Work out the finished part from the listing and answer in its coordinate system (mm). A direction names the side the tool comes from. Coordinates: 2 decimals unless noted, no trailing zeros. Order: outer loops, then holes, each group sorted by start corner. A loop starts at its lowest first (then second) coordinate and runs counter-clockwise, first axis right, second up.
1. A tool of negligible diameter and unlimited length cuts with its end or side. For faces 1 (the flat face through (4.445, 38, 11)), 2 (the flat face through (-8.255, 38, 11)), 3 (the flat face through (6.377, -26.854, 11.001)), 4 (the flat face through (8.255, 38, 11)), from which of +Z, -Z, +X, -X, +Y, -Y can it reach the whole face along a straight path? Write none if from no direction.
2. The part is cut by section B-B, the plane y = -26. Give the vertices of the cut face in (x, z) (3 decimals).
3. Flat-ended cylindrical pins translate along their axes: pin 1 Ø6 at (y, z) = (-31.5, 15) entering from -X (3 decimals); pin 2 Ø8 at (y, z) = (36.5, 20) entering from +X (3 decimals); pin 3 Ø7.5 at (x, y) = (3.5, 6) entering from +Z (3 decimals). Find the tip coordinate at first contact, or state that the pin passes through.
4. Find the intervals of material crossed by probe 1 along Z at (x, y) = (5.3, 38.1); probe 2 along X at (y, z) = (-46, 15) (3 decimals); probe 3 along Z at (x, y) = (11.75, -32.5) (3 decimals), in increasing order.
5. The part is cut by section D-D, the plane x = -2.25. Give the vertices of the cut face in (y, z) (3 decimals).
6. The part is cut by section C-C, the plane z = 13.25. Give the vertices of the cut face in (x, y) (3 decimals), then the cut area to 3 significant figures.
7. Determine the mould class of faces 5 (the cylindrical face through (11.172, 62.051, 1.61)), 6 (the flat face through (8.255, -38, 11)), 7 (the cylindrical face through (6.38, 37.99, 22.86)) for opening direction Y: +Y half, -Y half, draft (parallel to the pull), parting line (faces both ways), or undercut.
8. The part is cut by section A-A, the plane z = 8. Give the vertices of the cut face in (x, y) (3 decimals).
```python
from build123d import *

# Parameters (mm, degrees)
F0_W     = 25.4
F0_H     = 127
F1_DEPTH = 3.175
F3_DEPTH = 8.255
F4_DEPTH = 4.445
F5_R     = 0.9
F6_DEPTH = 20.956
F7_R     = 5.08


# Not quite as in the source:
# - a pattern or mirror of a feature is missing from the dataset's text; its kind, count and spacing are read off the source's solid


with BuildPart() as f1:
    # F0 (on Top) → F1 (new body)
    with BuildSketch(Plane.XY):
        Rectangle(F0_W, F0_H)
    extrude(amount=F1_DEPTH)

    # F2 (on Right) → F3 (join, symmetric)
    with BuildSketch(Plane.YZ):
        with BuildLine():
            Line((-44.6991135768, 19.05), (-53.8645491002, 3.175))
            Line((-53.8645491002, 3.175), (-22.3354508998, 3.175))
            Line((-22.3354508998, 3.175), (-31.5008864232, 19.05))
            ThreePointArc((-31.5008864232, 19.05), (-38.1, 22.86), (-44.6991135768, 19.05))
        make_face()
    f3 = extrude(amount=F3_DEPTH, both=True)

    # F3_copies: F3 across plane
    add(f3.mirror(Plane.ZX))

    # F2 (on Right) → F4 (cut, symmetric)
    with BuildSketch(Plane.YZ):
        with BuildLine():
            Line((-44.6991135768, 19.05), (-53.8645491002, 3.175))
            Line((-53.8645491002, 3.175), (-22.3354508998, 3.175))
            Line((-22.3354508998, 3.175), (-31.5008864232, 19.05))
            ThreePointArc((-31.5008864232, 19.05), (-38.1, 22.86), (-44.6991135768, 19.05))
        make_face()
    f4 = extrude(amount=F4_DEPTH, both=True, mode=Mode.SUBTRACT)

    # F4_copies: F4 across plane
    add(f4.mirror(Plane.ZX), mode=Mode.SUBTRACT)

    # F5 (on face) → F6 (cut, through all)
    with BuildSketch(Plane.YZ.offset(8.255)):
        with Locations((-38.1, 15.24)):
            Circle(F5_R)
    f6 = extrude(amount=-F6_DEPTH, mode=Mode.SUBTRACT)

    # F6_copies: F6 across plane
    add(f6.mirror(Plane.ZX), mode=Mode.SUBTRACT)

    # F7
    f7_edges = [f1.edges().sort_by_distance(p)[0] for p in [
        (12.7, -63.5, 1.5875),
        (-12.7, -63.5, 1.5875),
        (12.7, 63.5, 1.5875),
        (-12.7, 63.5, 1.5875),
    ]]
    fillet(f7_edges, radius=F7_R)


solid = f1.part
```
Geometry says:
1. face 1: +Z, +Y, -Y
1. face 2: +Z, -X, +Y, -Y
1. face 3: +Z, +X, -X
1. face 4: +Z, +X, +Y, -Y
2. outline: (-12.7, 0) - (12.7, 0) - (12.7, 3.175) - (8.255, 3.175) - (8.255, 9.522) - (4.445, 9.522) - (4.445, 3.175) - (-4.445, 3.175) - (-4.445, 9.522) - (-8.255, 9.522) - (-8.255, 3.175) - (-12.7, 3.175) - close
3. pin 1: stops at x = -8.255
3. pin 2: stops at x = 8.255
3. pin 3: stops at z = 3.175
4. probe 1: z = 0 to 14.34, 16.14 to 22.86
4. probe 2: x = -8.255 to -4.445, 4.445 to 8.255
4. probe 3: z = 0 to 3.175
5. outline: (-63.5, 0) - (63.5, 0) - (63.5, 3.175) - (-63.5, 3.175) - close
6. outline: (-8.255, -48.048) - (-4.445, -48.048) - (-4.445, -28.152) - (-8.255, -28.152) - close; (-8.255, 28.152) - (-4.445, 28.152) - (-4.445, 48.048) - (-8.255, 48.048) - close; (4.445, -48.048) - (8.255, -48.048) - (8.255, -28.152) - (4.445, -28.152) - close; (4.445, 28.152) - (8.255, 28.152) - (8.255, 48.048) - (4.445, 48.048) - close
6. area: 303 mm2
7. face 5: +Y half
7. face 6: draft
7. face 7: undercut
8. outline: (-8.255, -51.079) - (-4.445, -51.079) - (-4.445, -25.121) - (-8.255, -25.121) - close; (-8.255, 25.121) - (-4.445, 25.121) - (-4.445, 51.079) - (-8.255, 51.079) - close; (4.445, -51.079) - (8.255, -51.079) - (8.255, -25.121) - (4.445, -25.121) - close; (4.445, 25.121) - (8.255, 25.121) - (8.255, 51.079) - (4.445, 51.079) - close
